Autodesk Inventor part; units mm, degrees
ref_plane "YZ Plane" through (0, 0, 0) normal (1, 0, 0) x (0, 1, 0)
ref_plane "XZ Plane" through (0, 0, 0) normal (0, 1, 0) x (-1, 0, 0)
ref_plane "XY Plane" through (0, 0, 0) normal (0, 0, 1) x (1, 0, 0)
sketch "Sketch1" plane through (0, 0, 0) normal (0, 1, 0) x (-1, 0, 0)
  line L0 (-4.1, 2.85) -> (-3.1, 2.85)
  line L1 (-3.1, 2.85) -> (-3.1, 2.35)
  line L2 (-3.1, 2.35) -> (2.5, 2.35)
  line L3 (2.5, 2.35) -> (2.5, -2.35)
  line L4 (-4.1, 2.85) -> (-3.6981, 4.35)
  line L5 (-3.6981, 4.35) -> (-7.6981, 4.35)
  line L6 (-7.6981, 4.35) -> (-7.6981, 2.35)
  line L7 (-7.6981, 2.35) -> (-20.6981, 2.35)
  line L8 (-20.6981, 2.35) -> (-21.6981, 1.35)
  line L9 (-21.6981, 1.35) -> (-21.6981, -0.65)
  line L10 (-21.6981, -0.65) -> (-19.966, -1.65)
  line L11 (-19.966, -1.65) -> (-7.6981, -1.65)
  line L12 (-7.6981, -1.65) -> (-7.6981, -3.25)
  line L13 (-7.6981, -3.25) -> (-3.9124, -3.25)
  line L14 (-3.9124, -3.25) -> (-4.1, -2.55)
  line L15 (-4.1, -2.55) -> (-3.6, -2.55)
  line L16 (-3.6, -2.55) -> (-3.6, -2.35)
  line L17 (-3.6, -2.35) -> (2.5, -2.35)
  circle A0 centre (0, 0) radius 1.4
  dimension "d1" = 4
  dimension "d2" = 2
  dimension "d3" = 75
  dimension "d4" = 4.7
  dimension "d5" = 5.6
  dimension "d6" = 1
  dimension "d7" = 0.5
  dimension "d8" = 75
  dimension "d9" = 7.6
  dimension "d10" = 2
  dimension "d11" = 0.5
  dimension "d12" = 0.2
  dimension "d13" = 2.8
  dimension "d14" = 2.5
  dimension "d15" = 2.35
  dimension "d17" = 0
  dimension "d18" = 0
  dimension "d19" = 4
  dimension "d20" = 0
  dimension "d21" = 0
  dimension "d23" = 2
  dimension "d24" = 60
  dimension "d25" = 45
  dimension "d26" = 14
  dimension "d27" = 1
extrude "Plate1" add sketch "Sketch1" along normal blind 1
chamfer "Corner Chamfer1" distance 1 angle 45 2 edges at (-2.5, 0.5, 2.35) (-2.5, 0.5, -2.35)
equation "\"d8\" = d3"
equation "\"d15\" = 0.5 * d4"
equation "\"d31\" = Thickness"
equation "\"BendRadius\" = Thickness"
equation "\"BendReliefWidth\" = Thickness"
equation "\"BendReliefDepth\" = 0.5 * Thickness"
equation "\"CornerReliefSize\" = 4 * Thickness"
equation "\"MinimumRemnant\" = 2 * Thickness"
equation "\"TransitionRadius\" = BendRadius"
equation "\"JacobiRadiusSize\" = BendRadius"
equation "\"GapSize\" = Thickness"
equation "\"d16\" = BendRadius"
properties part number "PlacaTerraPlug" material "Steel, Galvanized"
Design review of the part built by this model. Coordinates are the model's own, in mm. A direction names the side the tool comes from. Give positions to 0.01 mm unless a question says otherwise; leave off trailing zeros. Order: outer loops, then holes, each group sorted by start corner. A loop starts at its lowest first (then second) coordinate and runs counter-clockwise, first axis right, second up.
1. For pin 1 Ø0.5 at (x, y) = (2, 0.5) entering from -Z; pin 2 Ø2.5 at (x, z) = (0, 0) entering from +Y; pin 3 Ø0.5 at (x, y) = (0, 0.5) entering from +Z, all flat-tipped, find the tip position at first contact; note any pin that passes through.
Solution:
pin 1: stops at z = -2.35
pin 2: passes through
pin 3: stops at z = 2.35
2. Add section A-A, the plane z = 0. State the section outline as (x, y) points, then the cut area to 3 significant figures.
Solution:
outline: (-2.5, 0) - (-1.4, 0) - (-1.4, 1) - (-2.5, 1) - close; (1.4, 0) - (21.7, 0) - (21.7, 1) - (1.4, 1) - close
area: 21.4 mm2
3. Add section B-B, the plane x = 0. State the section outline as (y, z) points, then the cut area to 3 significant figures.
Solution:
outline: (0, -2.35) - (1, -2.35) - (1, -1.4) - (0, -1.4) - close; (0, 1.4) - (1, 1.4) - (1, 2.35) - (0, 2.35) - close
area: 1.90 mm2
4. Add section C-C, the plane y = 0.25. State the section outline as (x, z) points, then the cut area to 3 significant figures.
Solution:
outline: (-2.5, -1.35) - (-1.5, -2.35) - (3.6, -2.35) - (3.6, -2.55) - (4.1, -2.55) - (3.91, -3.25) - (7.7, -3.25) - (7.7, -1.65) - (19.97, -1.65) - (21.7, -0.65) - (21.7, 1.35) - (20.7, 2.35) - (7.7, 2.35) - (7.7, 4.35) - (3.7, 4.35) - (4.1, 2.85) - (3.1, 2.85) - (3.1, 2.35) - (-1.5, 2.35) - (-2.5, 1.35) - close; hole circle Ø2.8 at (0, 0)
area: 107 mm2
5. Mouldability with a two-part tool opening along Z and no side actions: class faces 1 (the flat face through (3.9, 0.5, 3.6)), 2 (the flat face through (7.698, 0.5, 3.4)), 3 (the flat face through (13.9, 0.5, -1.65)) as +Z half, -Z half, draft (parallel to the pull), parting line (faces both ways), or undercut.
Solution:
face 1: undercut
face 2: draft
face 3: -Z half
6. To check wall thickness, follow L1, parallel to Z at x = 0, y = 0.7; L2, parallel to Z at x = 13.5, y = 0.9; L3, parallel to X at y = 0.1, z = 0.5. State the ranges of each line that lie inside material, in increasing order.
Solution:
L1: z = -2.35 to -1.4, 1.4 to 2.35
L2: z = -1.65 to 2.35
L3: x = -2.5 to -1.31, 1.31 to 21.7
7. Add section D-D, the plane x = 13.25. State the section outline as (y, z) points.
Solution:
outline: (0, -1.65) - (1, -1.65) - (1, 2.35) - (0, 2.35) - close
8. Tool access review of faces 4 (the flat face through (14.1, 0.5, 2.35)), 5 (the flat face through (3.6, 0.5, 2.85)), 6 (the flat face through (1.1, 0.5, -2.35)), 7 (the flat face through (7.698, 0.5, -2.4)): name each direction out of +Z, -Z, +X, -X, +Y, -Y from which nothing blocks a thin tool from reaching the whole face with its end or side.
Solution:
face 4: +Z, +X, +Y, -Y
face 5: -X, +Y, -Y
face 6: -Z, -X, +Y, -Y
face 7: -Z, +X, +Y, -Y
